from build123d import *

# Parameters (mm, degrees)
SKETCH1_R           = 3
BOSS_EXTRUDE1_DEPTH = 2


# Read off the part's stored shape, not the designer's step: Cut-Extrude2
with BuildPart() as part:
    # Sketch1 → Boss-Extrude1 (new body)
    with BuildSketch(Plane(origin=(0, 0, 0), x_dir=(1, 0, 0), z_dir=(0, 1, 0))):
        Polygon((0, -5.773502692), (5, -2.886751346), (5, 2.886751346), (0, 5.773502692), (-5, 2.886751346), (-5, -2.886751346), align=None)
        with Locations(Location((0, 0, 0), (0, 0, 270))):
            Circle(SKETCH1_R, mode=Mode.SUBTRACT)
    extrude(amount=BOSS_EXTRUDE1_DEPTH)

    # Cut-Extrude2 outline → Cut-Extrude2 (revolve, cut)
    with BuildSketch(Plane.XY):
        Polygon((5.773502708, 2), (5, 2), (5.773502708, 1.350954163), align=None)
    revolve(axis=Axis((0, 0, 0), (0, 1, 0)), mode=Mode.SUBTRACT)


solid = part.part
Can you work these out from the model? Positions are in its coordinate system, mm. Round coordinates to 2 decimals unless told otherwise and drop trailing zeros. Loops run counter-clockwise (first coordinate to the right, second up) from the corner with the lowest first, then second, coordinate; pieces in that order, holes last. Notation, with made-up numbers: (26.5, 18.25) - (32.5, 18.25) arc R11 cw to (32.5, 33.25) - close; hole circle Ø8 at (-19, 54). An arc over 180 degrees is marked (long way). Answer in a Markdown table with one row per item. Add a question column.
Q1. We'd pull the mould along X, two halves only. Please class faces 1 (the flat face through (5, 1, 0)), 2 (the conical face through (-4.499, 1.842, 2.583)), 3 (the flat face through (-2.3, 0, 2.5)), 4 (the cylindrical face through (0.9, 0.99, 2.86)): pulls with the +X half, pulls with the -X half, needs draft (parallel to the pull), parting line crosses it, or undercut.
Q2. I need wall thicknesses on L1, parallel to X at y = 1.25, z = 0; L2, parallel to X at y = 0.5, z = -2.5; L3, parallel to Z at x = -2.5, y = 1.2. Which ranges of each line are inside material? Lowest first, please.
Q3. I want a section at A-A on y = 1.55. List the corners of the cut face in (x, z) for me.
A:
| question | item | result |
|---|---|---|
| 1 | face 1 | pulls with the +X half |
| 1 | face 2 | pulls with the -X half |
| 1 | face 3 | needs draft |
| 1 | face 4 | undercut |
| 2 | L1 | -5 to -3, 3 to 5 |
| 2 | L2 | -5 to -1.66, 1.66 to 5 |
| 2 | L3 | -4.33 to -1.66, 1.66 to 4.33 |
| 3 | outline | (-5, -2.38) arc R5.54 ccw to (-4.56, -3.14) - (-0.44, -5.52) arc R5.54 ccw to (0.44, -5.52) - (4.56, -3.14) arc R5.54 ccw to (5, -2.38) - (5, 2.38) arc R5.54 ccw to (4.56, 3.14) - (0.44, 5.52) arc R5.54 ccw to (-0.44, 5.52) - (-4.56, 3.14) arc R5.54 ccw to (-5, 2.38) - close; hole circle Ø6 at (0, 0) |
